Can you work these out from the model? Positions are in its coordinate system, mm. A direction names the side the tool comes from. Round coordinates to 2 decimals unless told otherwise and drop trailing zeros. Loops run counter-clockwise (first coordinate to the right, second up) from the corner with the lowest first, then second, coordinate; pieces in that order, holes last. Notation, with made-up numbers: (25, -22.5) - (63, -22.5) arc R26 ccw to (63, -8.5) - close; hole circle Ø11 at (51, -2.5). An arc over 180 degrees is marked (long way). Answer as CSV lines item,"result".
```python
from build123d import *

# Parameters (mm, degrees)
SKETCH_1_W          = 17
SKETCH_1_H          = 12
EXTRUDE_1_DEPTH     = 4.6
SKETCH_3_W          = 17
SKETCH_3_H          = 5
CUT_EXTRUDE_1_DEPTH = 2.6
SKETCH_4_R          = 1
CUT_EXTRUDE_2_DEPTH = 2


with BuildPart() as part:
    # 스케치1 → 보스-돌출1 (new body)
    with BuildSketch(Plane(origin=(0, 0, 0), x_dir=(1, 0, 0), z_dir=(0, 1, 0))):
        Rectangle(SKETCH_1_W, SKETCH_1_H)
    extrude(amount=EXTRUDE_1_DEPTH)

    # 스케치3 → 컷-돌출1 (cut)
    with BuildSketch(Plane(origin=(0, 2.6, 0), x_dir=(1, 0, 0), z_dir=(0, 1, 0))):
        Rectangle(SKETCH_3_W, SKETCH_3_H)
    extrude(amount=-CUT_EXTRUDE_1_DEPTH, mode=Mode.SUBTRACT)

    # 스케치4 → 컷-돌출2 (cut)
    with BuildSketch(Plane(origin=(0, 4.6, 0), x_dir=(1, 0, 0), z_dir=(0, 1, 0))):
        with Locations((0, 4)):
            Circle(SKETCH_4_R)
        with Locations((0, -4)):
            Circle(SKETCH_4_R)
    extrude(amount=-CUT_EXTRUDE_2_DEPTH, mode=Mode.SUBTRACT)


solid = part.part
```
Q1. I'm going to push a flat-ended pin straight in: pin 1 Ø0.6 at (x, z) = (0, -4) entering from +Y. Where does the tip first touch, or does it pass through?
Checks:
pin 1,"y = 2.6"
Q2. Imagine slicing it at C-C (y = 2.8). Write out the boundary of the cut face in (x, z).
Checks:
outline,"(-8.5, -6) - (8.5, -6) - (8.5, 6) - (-8.5, 6) - close; hole circle Ø2 at (0, -4); hole circle Ø2 at (0, 4)"
Q3. We'd pull the mould along X, two halves only. Please class faces 1 (the flat face through (8.5, 3, 0)), 2 (the flat face through (0, 2.6, 4)), 3 (the flat face through (0, 1, -2.5)): pulls with the +X half, pulls with the -X half, needs draft (parallel to the pull), parting line crosses it, or undercut.
Checks:
face 1,"pulls with the +X half"
face 2,"undercut"
face 3,"needs draft"
Q4. Imagine slicing it at B-B (z = -4). Write out the boundary of the cut face in (x, y).
Checks:
outline,"(-8.5, 0) - (8.5, 0) - (8.5, 4.6) - (1, 4.6) - (1, 2.6) - (-1, 2.6) - (-1, 4.6) - (-8.5, 4.6) - close"
Q5. Imagine slicing it at A-A (x = 7.25). Write out the boundary of the cut face in (y, z).
Checks:
outline,"(0, -6) - (4.6, -6) - (4.6, 6) - (0, 6) - (0, 2.5) - (2.6, 2.5) - (2.6, -2.5) - (0, -2.5) - close"
Q6. If I drill on line 1 along Z through (x, y) = (0, 3.6); line 2 along X through (y, z) = (3, 4); line 3 along Z through (x, y) = (-4.25, 0.75), over which ranges is the centre line in solid material (lowest first)? Write a range as [from, to].
Checks:
line 1,"[-6, -5], [-3, 3], [5, 6]"
line 2,"[-8.5, -1], [1, 8.5]"
line 3,"[-6, -2.5], [2.5, 6]"
Q7. On a 3-axis mill with a long thin cutter (end or side, diameter ignored), from which of +Z, -Z, +X, -X, +Y, -Y can I reach the whole of each face in a straight line? I mean faces 4 (the cylindrical face through (0, 4, -5)), 5 (the flat face through (0, 1, 2.5)), 6 (the flat face through (0, 4.6, 0)). Say none if no direction works.
Checks:
face 4,"+Y"
face 5,"+X, -X, -Y"
face 6,"+Z, -Z, +X, -X, +Y"
Q8. Imagine slicing it at D-D (x = 0). Write out the boundary of the cut face in (y, z).
Checks:
outline,"(0, -6) - (4.6, -6) - (4.6, -5) - (2.6, -5) - (2.6, -3) - (4.6, -3) - (4.6, 3) - (2.6, 3) - (2.6, 5) - (4.6, 5) - (4.6, 6) - (0, 6) - (0, 2.5) - (2.6, 2.5) - (2.6, -2.5) - (0, -2.5) - close"
